CAD build for the part. Positions are in the model's coordinates, mm. A direction names the side the tool comes from. Coordinates: 2 decimals unless noted, no trailing zeros. Loops run counter-clockwise (first coordinate to the right, second up) from the corner with the lowest first, then second, coordinate; pieces in that order, holes last. Notation, with made-up numbers: (84.25, 6.25) -> (135.25, 6.25) arc R35 cw to (135.25, 45.25) -> close; hole circle Ø9 at (42, -22.5). An arc over 180 degrees is marked (long way). Return JSON: item names as keys, results as strings. Group by question number.
(1) Tool access for faces 1 (the face through (2.4, -4.1, -2.5)), 2 (the face through (6, 0, -2)), 3 (the face through (-1, 6, -4)): list every direction of +Z, -Z, +X, -X, +Y, -Y with a clear straight run to the whole face (end or side of a thin tool).
(2) Probe L1, parallel to Y at x = 0, z = 3.55; L2, parallel to Z at x = -1.5, y = -3; L3, parallel to Y at x = -1, z = 2. List the from-to ranges inside material, lowest first.
(3) Saw through at D-D on z = -1. Write the cut outline in (x, y).
(4) Flat gauge pins, fed straight in: pin 1 Ø1.4 at (x, z) = (5.5, -3.5) entering from -Y; pin 2 Ø6 at (x, z) = (5, -2) entering from -Y; pin 3 Ø0.9 at (x, y) = (0.5, -5.5) entering from -Z. Where does each tip first touch, or does it go through?
(5) Saw through at A-A on z = -2.5. Write the cut outline in (x, y), then the cut area to 3 significant figures.
(6) Saw through at B-B on y = 0. Write the cut outline in (x, z), then the cut area to 3 significant figures.
(7) Saw through at C-C on x = 0.25. Write the cut outline in (y, z), then the cut area to 3 significant figures.
```python
from build123d import *

# Parameters (mm, degrees)
F0_R     = 6.5
F0_R_2   = 4.75
F1_DEPTH = 5
F0_R_3   = 2.5
F2_DEPTH = 5
F3_W     = 1.8564560947
F3_H     = 2
F3_W_2   = 2
F3_H_2   = 1.8564560947
F4_DEPTH = 3
F6_DEPTH = 5


with BuildPart() as f1:
    # F0 (on Top) → F1 (new body)
    with BuildSketch(Plane.XY):
        Circle(F0_R)
        Circle(F0_R_2, mode=Mode.SUBTRACT)
    extrude(amount=-F1_DEPTH)

    # F0 (on Top) → F2 (join)
    with BuildSketch(Plane.XY):
        Circle(F0_R)
        Circle(F0_R_2, mode=Mode.SUBTRACT)
        Circle(F0_R_2)
        Circle(F0_R_3, mode=Mode.SUBTRACT)
    extrude(amount=F2_DEPTH)

    # F3 (on face) → F4 (cut)
    with BuildSketch(Plane(origin=(0, 0, -5), x_dir=(1, 0, 0), z_dir=(0, 0, -1))):
        with Locations((-5.5717719526, 0)):
            Rectangle(F3_W, F3_H)
        with Locations((0, -5.5717719526)):
            Rectangle(F3_W_2, F3_H_2)
        with Locations((5.5717719526, 0)):
            Rectangle(F3_W, F3_H)
        with Locations((0, 5.5717719526)):
            Rectangle(F3_W_2, F3_H_2)
    extrude(amount=-F4_DEPTH, mode=Mode.SUBTRACT)

    # F5 (on face) → F6 (cut, through all)
    with BuildSketch(Plane.XY):
        Polygon((0.0516711998, -5.1958955039), (4.5256131017, -2.5531991802), (4.4739419018, 2.6426963236), (-0.0516711998, 5.1958955039), (-4.5256131017, 2.5531991802), (-4.4739419018, -2.6426963236), align=None)
    extrude(amount=-F6_DEPTH, mode=Mode.SUBTRACT)


solid = f1.part
```
Geometry results:
{
 "1": {"face 1": "-Z", "face 2": "-Z, +X, -X", "face 3": "-Z, +Y, -Y"},
 "2": {"L1": "-6.5 to -2.5, 2.5 to 6.5", "L2": "0 to 5", "L3": "-6.42 to -2.29, 2.29 to 6.42"},
 "3": {"outline": "circle Ø13 at (0, 0); hole (-4.53, 2.55) -> (-4.51, 1.48) arc R4.75 ccw to (-4.48, -1.57) -> (-4.47, -2.64) -> (-3.54, -3.17) arc R4.75 ccw to (-0.89, -4.67) -> (0.05, -5.2) -> (0.98, -4.65) arc R4.75 ccw to (3.6, -3.1) -> (4.53, -2.55) -> (4.51, -1.48) arc R4.75 ccw to (4.48, 1.57) -> (4.47, 2.64) -> (3.54, 3.17) arc R4.75 ccw to (0.89, 4.67) -> (-0.05, 5.2) -> (-0.98, 4.65) arc R4.75 ccw to (-3.6, 3.1) -> close"},
 "4": {"pin 1": "y = -4.38", "pin 2": "y = -6.18", "pin 3": "z = -2"},
 "5": {"outline": "(-6.42, -1) arc R6.5 ccw to (-1, -6.42) -> (-1, -4.64) arc R4.75 cw to (-3.54, -3.17) -> (-4.47, -2.64) -> (-4.48, -1.57) arc R4.75 cw to (-4.64, -1) -> close; (-6.42, 1) -> (-4.64, 1) arc R4.75 cw to (-4.51, 1.48) -> (-4.53, 2.55) -> (-3.6, 3.1) arc R4.75 cw to (-1, 4.64) -> (-1, 6.42) arc R6.5 ccw to start; (1, -6.42) arc R6.5 ccw to (6.42, -1) -> (4.64, -1) arc R4.75 cw to (4.51, -1.48) -> (4.53, -2.55) -> (3.6, -3.1) arc R4.75 cw to (1, -4.64) -> close; (1, 4.64) arc R4.75 cw to (3.54, 3.17) -> (4.47, 2.64) -> (4.48, 1.57) arc R4.75 cw to (4.64, 1) -> (6.42, 1) arc R6.5 ccw to (1, 6.42) -> close", "area": "46.2 mm²"},
 "6": {"outline": "(-6.5, -2) -> (-4.75, -2) -> (-4.75, 0) -> (-2.5, 0) -> (-2.5, 5) -> (-6.5, 5) -> close; (2.5, 0) -> (4.75, 0) -> (4.75, -2) -> (6.5, -2) -> (6.5, 5) -> (2.5, 5) -> close", "area": "47.0 mm²"},
 "7": {"outline": "(-6.5, -2) -> (-5.08, -2) -> (-5.08, 0) -> (-2.49, 0) -> (-2.49, 5) -> (-6.5, 5) -> close; (2.49, 0) -> (5.03, 0) -> (5.03, -2) -> (6.5, -2) -> (6.5, 5) -> (2.49, 5) -> close", "area": "45.8 mm²"}
}
